```python
from build123d import *

# Parameters (mm, degrees)
F0_W     = 33.02
F0_H     = 68.58
F1_DEPTH = 22.86
F2_R     = 3.81
F3_W     = 3.073085
F3_H     = 3.073089
F4_DEPTH = 4.572


with BuildPart() as f1:
    # F0 (on Front) → F1 (new body)
    with BuildSketch(Plane.XZ):
        with Locations((16.51, 34.29)):
            Rectangle(F0_W, F0_H)
    extrude(amount=F1_DEPTH)

    # F2
    f2_edges = [f1.edges().sort_by_distance(p)[0] for p in [
        (33.02, -22.86, 34.29),
        (33.02, -11.43, 68.58),
        (16.51, -22.86, 68.58),
        (0, -22.86, 34.29),
        (16.51, -22.86, 0),
        (33.02, -11.43, 0),
        (33.02, 0, 34.29),
        (16.51, 0, 0),
        (0, 0, 34.29),
        (0, -11.43, 68.58),
        (0, -11.43, 0),
        (16.51, 0, 68.58),
    ]]
    fillet(f2_edges, radius=F2_R)

    # F3 (on face) → F4 (join)
    with BuildSketch(Plane.XZ.offset(22.86)):
        with Locations((9.438765, 60.034938)):
            Rectangle(F3_W, F3_H)
    extrude(amount=F4_DEPTH)


solid = f1.part
```
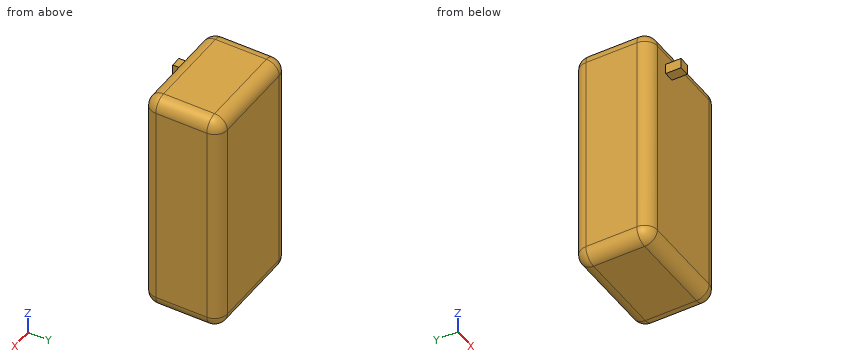
Build history of the part. All positions in model axes, mm. Round coordinates to 2 decimals unless told otherwise and drop trailing zeros. Write each loop counter-clockwise with the first axis right and the second up, starting at its lowest first coordinate (ties: lowest second). Pieces come first, ordered by that corner, then holes.
1) Band-saw the part on B-B, the plane x = 9.5. List the corners of the cut face in (y, z).
2) Drill centre lines: probe 1 along Z at (x, y) = (18, -3.5); probe 2 along Y at (x, z) = (18, 32); probe 3 along Y at (x, z) = (28, 3.5). Where is each one in solid material? Low to high.
3) Band-saw the part on D-D, the plane y = -25.25. List the corners of the cut face in (x, z).
4) Band-saw the part on C-C, the plane y = -21.5. List the corners of the cut face in (x, z).
5) Pin check, flat tips, straight feed: pin 1 (3.5 mm diameter, centred on x = 8.5, y = -26, fed in from +Z); pin 2 (0.9 mm diameter, centred on y = -25, z = 60.5, fed in from +X); pin 3 (3.5 mm diameter, centred on x = 10, y = -26, fed in from -Z). Stop position of each tip, or through.
6) Band-saw the part on A-A, the plane z = 17. List the corners of the cut face in (x, y), and give its area (3 significant figures).
Ans:
1. outline: (-27.43, 58.5) - (-22.86, 58.5) - (-22.86, 3.81) arc R3.81 ccw to (-19.05, 0) - (-3.81, 0) arc R3.81 ccw to (0, 3.81) - (0, 64.77) arc R3.81 ccw to (-3.81, 68.58) - (-19.05, 68.58) arc R3.81 ccw to (-22.86, 64.77) - (-22.86, 61.57) - (-27.43, 61.57) - close
2. probe 1: z = 0.01 to 68.57
2. probe 2: y = -22.86 to 0
2. probe 3: y = -22.85 to -0.01
3. outline: (7.9, 58.5) - (10.98, 58.5) - (10.98, 61.57) - (7.9, 61.57) - close
4. outline: (0.89, 3.81) arc R2.92 ccw to (3.81, 0.89) - (29.21, 0.89) arc R2.92 ccw to (32.13, 3.81) - (32.13, 64.77) arc R2.92 ccw to (29.21, 67.69) - (3.81, 67.69) arc R2.92 ccw to (0.89, 64.77) - close
5. pin 1: stops at z = 61.57
5. pin 2: stops at x = 10.98
5. pin 3: stops at z = 58.5
6. outline: (0, -19.05) arc R3.81 ccw to (3.81, -22.86) - (29.21, -22.86) arc R3.81 ccw to (33.02, -19.05) - (33.02, -3.81) arc R3.81 ccw to (29.21, 0) - (3.81, 0) arc R3.81 ccw to (0, -3.81) - close
6. area: 742 mm2
